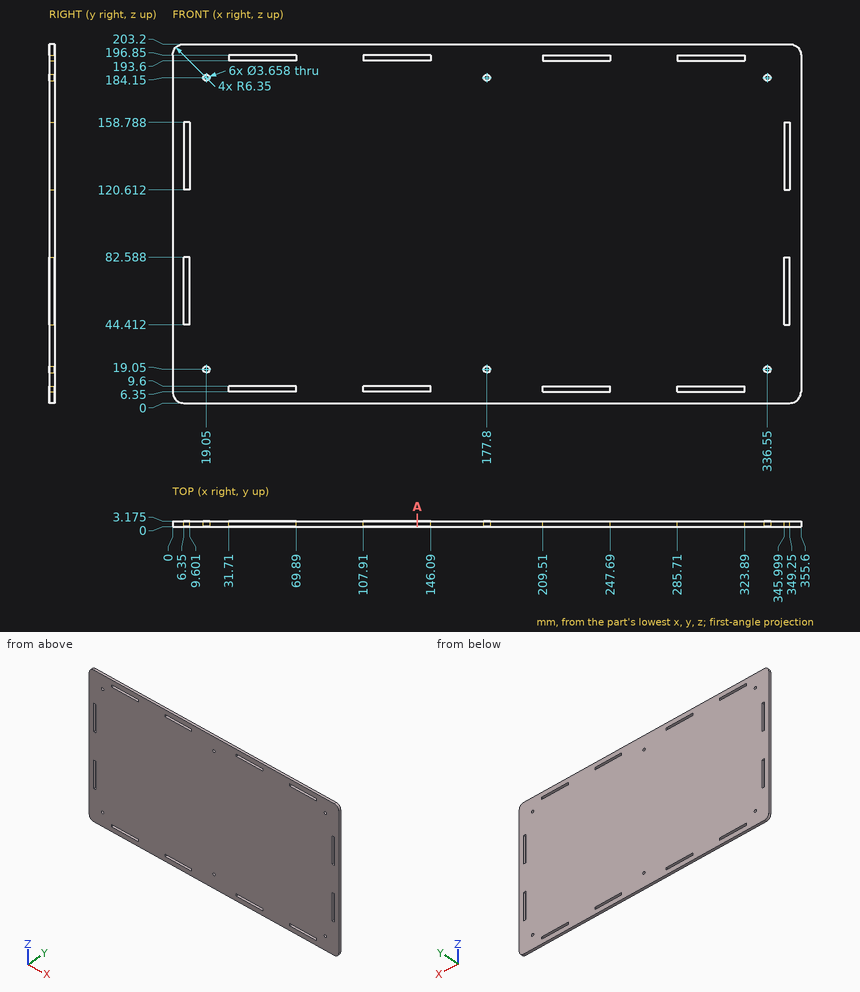
Part print with two shaded views. Sizes in mm from the minimum x, y, z corner. Give positions to 0.01 mm unless a question says otherwise; leave off trailing zeros.
1) Pin check, flat tip, straight feed: pin 1 (2 mm diameter, centred on x = 269.5, z = 46, fed in from -Y). Stop position of the tip, or through.
2) Saw through at A-A, the plane x = 138.5. Count the separate pieces of the cut face and the enclosed holes in it.
3) Wall check: probe 1 along X at (y, z) = (2.2, 19.05); probe 2 along Z at (x, y) = (19.05, 2.45); probe 3 along X at (y, z) = (2.45, 72). Give the ranges that are in metal, low to high.
Computed:
1. pin 1: stops at y = 0
2. separate pieces: 3
2. enclosed holes: 0
3. probe 1: x = 0 to 17.22, 20.88 to 175.97, 179.63 to 334.72, 338.38 to 355.6
3. probe 2: z = 0 to 17.22, 20.88 to 182.32, 185.98 to 203.2
3. probe 3: x = 0 to 6.35, 9.6 to 346, 349.25 to 355.6
